from build123d import *

# Parameters (mm, degrees)
P_IDAT_VYSUNUT_M1_DEPTH  = 0.8
SKICA2_R                 = 1
ODEBRAT_VYSUNUT_M1_DEPTH = 94.955095657
SKICA3_R                 = 0.75
ODEBRAT_VYSUNUT_M2_DEPTH = 94.955095657
SKICA8_R                 = 1.5
ODEBRAT_VYSUNUT_M4_DEPTH = 94.955095657


with BuildPart() as part:
    # Skica1 → Přidat vysunutím1 (new, symmetric)
    with BuildSketch(Plane(origin=(0, 0, 0), x_dir=(1, 0, 0), z_dir=(0, 1, 0))):
        with BuildLine():
            Line((-25, 15), (25, 15))
            ThreePointArc((25, 15), (28.535533906, 13.535533906), (30, 10))
            Line((30, 10), (30, -20))
            ThreePointArc((30, -20), (32.752551286, -28.660254038), (40, -34.142135624))
            Line((40, -34.142135624), (40, -61.846584384))
            ThreePointArc((40, -61.846584384), (36.172150801, -73.613552493), (26.153846154, -80.876302656))
            ThreePointArc((26.153846154, -80.876302656), (0, -85), (-26.153846154, -80.876302656))
            ThreePointArc((-26.153846154, -80.876302656), (-36.172150801, -73.613552493), (-40, -61.846584384))
            Line((-40, -61.846584384), (-40, -34.142135624))
            ThreePointArc((-40, -34.142135624), (-32.752551286, -28.660254038), (-30, -20))
            Line((-30, -20), (-30, 10))
            ThreePointArc((-30, 10), (-28.535533906, 13.535533906), (-25, 15))
        make_face()
    extrude(amount=P_IDAT_VYSUNUT_M1_DEPTH, both=True)

    # Skica2 → Odebrat vysunutím1 (cut, through all)
    with BuildSketch(Plane.XZ.offset(0.8)):
        with Locations(Location((-25.75, -9.25, 0), (0, 0, 270))):
            Circle(SKICA2_R)
        with Locations(Location((-25.75, 9.25, 0), (0, 0, 270))):
            Circle(SKICA2_R)
        with Locations(Location((25.75, 9.25, 0), (0, 0, 270))):
            Circle(SKICA2_R)
        with Locations(Location((25.75, -9.25, 0), (0, 0, 270))):
            Circle(SKICA2_R)
    extrude(amount=-ODEBRAT_VYSUNUT_M1_DEPTH, mode=Mode.SUBTRACT)

    # Skica3 → Odebrat vysunutím2 (cut, through all)
    with BuildSketch(Plane.XZ.offset(0.8)):
        with Locations(Location((-3.5, 4, 0), (0, 0, 270))):
            Circle(SKICA3_R)
        with Locations(Location((3.5, 4, 0), (0, 0, 270))):
            Circle(SKICA3_R)
        with Locations(Location((-3.5, -4, 0), (0, 0, 270))):
            Circle(SKICA3_R)
        with Locations(Location((3.5, -4, 0), (0, 0, 270))):
            Circle(SKICA3_R)
    extrude(amount=-ODEBRAT_VYSUNUT_M2_DEPTH, mode=Mode.SUBTRACT)

    # Skica8 → Odebrat vysunutím4 (cut, through all)
    with BuildSketch(Plane.XZ.offset(0.8)):
        with Locations(Location((18.5, 62, 0), (0, 0, 270))):
            Circle(SKICA8_R)
        with Locations(Location((-18.5, 62, 0), (0, 0, 270))):
            Circle(SKICA8_R)
    extrude(amount=-ODEBRAT_VYSUNUT_M4_DEPTH, mode=Mode.SUBTRACT)


solid = part.part
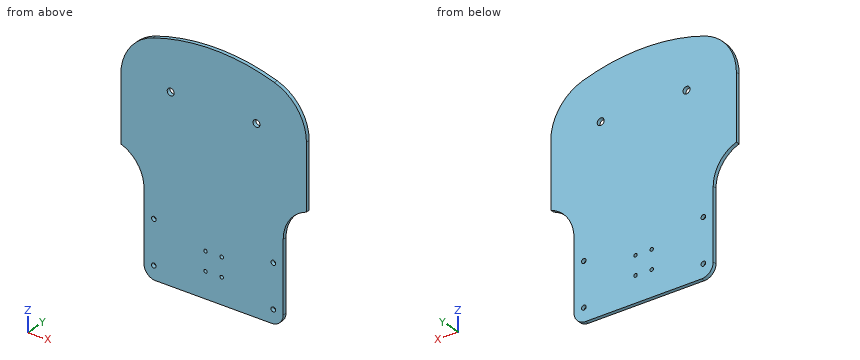
Can you work these out from the model? Positions are in its coordinate system, mm. Coordinates: 2 decimals unless noted, no trailing zeros. Write each loop counter-clockwise with the first axis right and the second up, starting at its lowest first coordinate (ties: lowest second). Pieces come first, ordered by that corner, then holes.
Q1. Imagine slicing it at B-B, the plane z = 18.5. List the corners of the cut face in (x, y) for me, plus the area to 3 significant figures.
Results found:
outline: (-30, -0.8) - (30, -0.8) - (30, 0.8) - (-30, 0.8) - close
area: 96.0 mm2
Q2. Imagine slicing it at A-A, the plane y = -0.1. Count the separate pieces of the cut face and the enclosed holes in it, plus the area to 3 significant figures.
Results found:
separate pieces: 1
enclosed holes: 10
area: 6,720 mm2
Q3. Imagine slicing it at C-C, the plane x = 22. List the corners of the cut face in (y, z) for me.
Results found:
outline: (-0.8, -15) - (0.8, -15) - (0.8, 82.1) - (-0.8, 82.1) - close
Q4. For P1, Ø0.9, axis at x = -3.5, z = 4, coming from the +Y side; P2, Ø2, axis at x = 3.5, z = 4, coming from the -Y side, each with a flat end and sliding along its axis, tell me the tip position at first contact or that it passes through.
Results found:
P1: passes through
P2: stops at y = -0.8
Q5. Please list where these lines run through material, in increasing order: L1, parallel to X at y = -0.2, z = -9.25; L2, parallel to X at y = -0.4, z = 4; L3, parallel to Z at x = -25.5, y = 0.05.
Results found:
L1: x = -30 to -26.75, -24.75 to 24.75, 26.75 to 30
L2: x = -30 to -4.25, -2.75 to 2.75, 4.25 to 30
L3: z = -14.97 to -10.22, -8.28 to 8.28, 10.22 to 81.08
